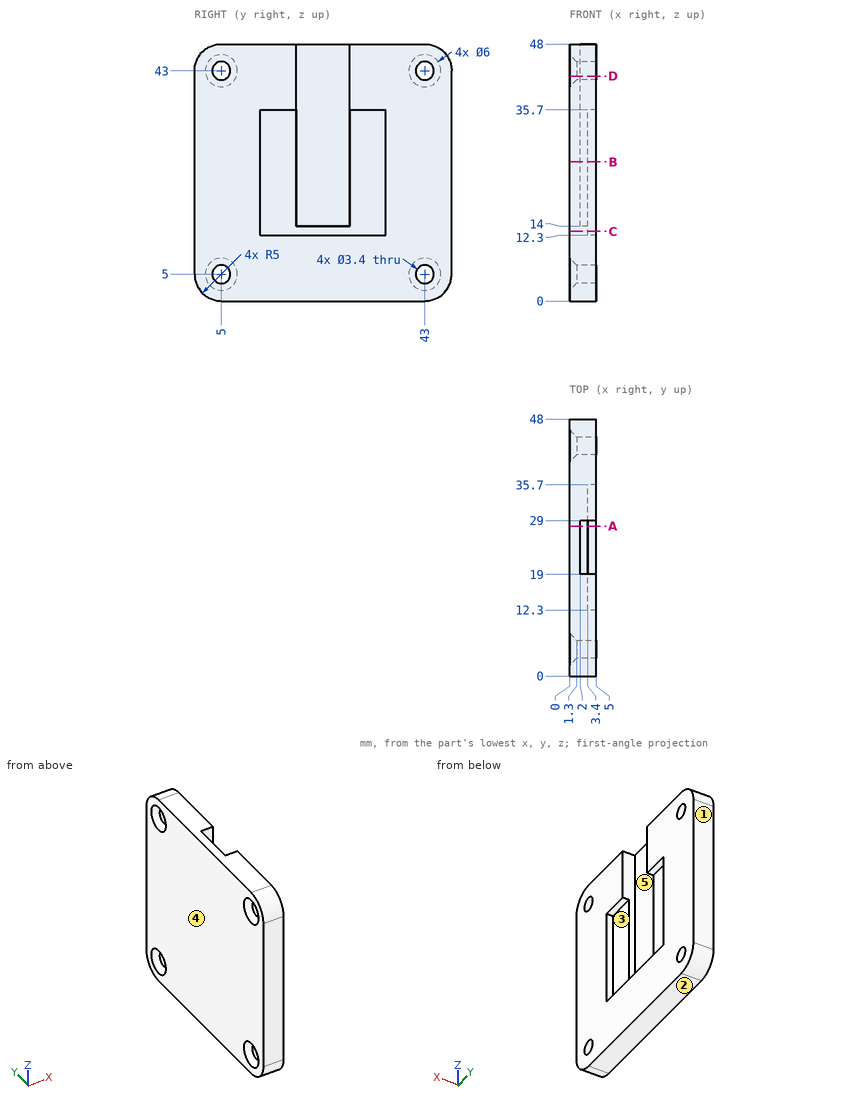
Design review of the part shown in the three views and the two pictorial views. Dimensions are in mm from the part's minimum x, y and z. A direction names the side the tool comes from. Coordinates: 2 decimals unless noted, no trailing zeros. Order: outer loops, then holes, each group sorted by start corner. A loop starts at its lowest first (then second) coordinate and runs counter-clockwise, first axis right, second up.
Item 1: Take a section at C-C, the plane z = 13. Write out the cut boundary in (x, y).
Item 2: The part is to be moulded in two halves that separate along Y. For the marked faces 1, 2 and 3, say which applies: pulls with the +Y half, pulls with the -Y half, needs draft (parallel to the pull), parting line crosses it, or undercut.
Item 3: For line 1 (Z direction, x = 3.4, y = 43); line 2 (Y direction, x = 4, z = 37.5); line 3 (Z direction, x = 3.6, y = 26.5), list the stretches that pass through material, from the lowest coordinate up.
Item 4: For the marked faces 4 and 5, list the 3-axis set-ups (+Z, -Z, +X, -X, +Y, -Y) from which the entire face can be reached by the end or side of a thin tool; tool diameter is ignored.
Item 5: For pin 1 Ø2.5 at (y, z) = (5, 5) entering from +X; pin 2 Ø0.8 at (x, y) = (4, 20.5) entering from +Z; pin 3 Ø4 at (y, z) = (43, 43) entering from -X; pin 4 Ø11 at (y, z) = (23.5, 31) entering from +X, all flat-tipped, find the tip position at first contact; note any pin that passes through.
Item 6: Take a section at D-D, the plane z = 42. Count the separate pieces of the cut face and the enclosed holes in it, then the cut area to 3 significant figures.
Item 7: Take a section at A-A, the plane y = 28. Write out the cut boundary in (x, z).
Item 8: Take a section at B-B, the plane z = 26. Write out the cut boundary in (x, y).
The answers:
1. outline: (0, 0) - (5, 0) - (5, 12.3) - (3.4, 12.3) - (3.4, 35.7) - (5, 35.7) - (5, 48) - (0, 48) - close
2. face 1: pulls with the +Y half
2. face 2: needs draft
2. face 3: undercut
3. line 1: z = 0 to 3.3, 6.7 to 41.3, 44.7 to 48
3. line 2: y = 0 to 19, 29 to 48
3. line 3: z = 0 to 12.3
4. face 4: +Z, -Z, -X, +Y, -Y
4. face 5: +Z, +X
5. pin 1: passes through
5. pin 2: stops at z = 12.3
5. pin 3: stops at x = 1
5. pin 4: stops at x = 3.4
6. separate pieces: 3
6. enclosed holes: 0
6. area: 179 mm2
7. outline: (0, 0) - (5, 0) - (5, 12.3) - (3.4, 12.3) - (3.4, 14) - (2, 14) - (2, 48) - (0, 48) - close
8. outline: (0, 0) - (5, 0) - (5, 12.3) - (3.4, 12.3) - (3.4, 19) - (2, 19) - (2, 29) - (3.4, 29) - (3.4, 35.7) - (5, 35.7) - (5, 48) - (0, 48) - close
